```python
from build123d import *

# Parameters (mm, degrees)
F0_W     = 101.6
F0_H     = 50.8
F1_DEPTH = 25.4
F2_W     = 50.8
F2_H     = 12.7
F4_DEPTH = 25.4
F3_W     = 25.4
F3_H     = 12.7
F5_DEPTH = 19.05
F6_R     = 6.35
F7_DEPTH = 101.6


with BuildPart() as f1:
    # F0 (on Front) → F1 (new body)
    with BuildSketch(Plane.XZ):
        Rectangle(F0_W, F0_H)
    extrude(amount=F1_DEPTH)

    # F2 (on face) → F4 (cut)
    with BuildSketch(Plane.XZ.offset(25.4)):
        with Locations((0.033422, 19.05)):
            Rectangle(F2_W, F2_H)
    extrude(amount=-F4_DEPTH, mode=Mode.SUBTRACT)

    # F3 (on face) → F5 (cut)
    with BuildSketch(Plane.YZ.offset(50.8)):
        with Locations((-12.7, -19.05)):
            Rectangle(F3_W, F3_H)
    extrude(amount=-F5_DEPTH, mode=Mode.SUBTRACT)

    # F6 (on face) → F7 (cut)
    with BuildSketch(Plane.YZ.offset(50.8)):
        with Locations((-12.7, 0)):
            Circle(F6_R)
    extrude(amount=-F7_DEPTH, mode=Mode.SUBTRACT)


solid = f1.part
```
Here's how the part is built. I have some questions about the finished solid (model axes, mm). A direction names the side the tool comes from. Coordinates: 2 decimals unless noted, no trailing zeros. Order: outer loops, then holes, each group sorted by start corner. A loop starts at its lowest first (then second) coordinate and runs counter-clockwise, first axis right, second up.
Item 1: Thinking about a two-plate mould opening in X: for faces 1 (the face through (0, -13, 12.7)), 2 (the face through (-50.8, -15.3, -6)), 3 (the face through (0.711, -6.643, 1.907)), 4 (the face through (-25.367, -13, 19)), which applies, pulls with the +X half, pulls with the -X half, needs draft (parallel to the pull), parting line crosses it, or undercut?
Response values:
face 1: undercut
face 2: pulls with the -X half
face 3: needs draft
face 4: undercut
Item 2: Which directions (+Z, -Z, +X, -X, +Y, -Y) give clear straight access to the entire face, cutting with the end or side of a thin tool? Please do faces 5 (the face through (41, -13, -12.7)), 6 (the face through (25.433, -13, 19)), 7 (the face through (50.8, -15.3, 6.1)).
Response values:
face 5: -Z, +X, +Y, -Y
face 6: +Z, +Y, -Y
face 7: +Z, -Z, +X, +Y, -Y
Item 3: If we section it at C-C, the plane x = 36.5: List the corners of the cut face in (y, z) for me, then the cut area to 3 significant figures.
Response values:
outline: (-25.4, -12.7) - (0, -12.7) - (0, 25.4) - (-25.4, 25.4) - close; hole circle Ø12.7 at (-12.7, 0)
area: 841 mm2
Item 4: If we section it at D-D, the plane y = -4.75: List the corners of the cut face in (x, z) for me.
Response values:
outline: (-50.8, -25.4) - (31.75, -25.4) - (31.75, -12.7) - (50.8, -12.7) - (50.8, 25.4) - (25.43, 25.4) - (25.43, 12.7) - (-25.37, 12.7) - (-25.37, 25.4) - (-50.8, 25.4) - close
Item 5: I'm going to push a flat-ended pin straight in: pin 1 Ø7.5 at (x, y) = (-3.5, -14.5) entering from +Z. Where does the tip first touch, or does it pass through?
Response values:
pin 1: stops at z = 12.7
Item 6: If we section it at A-A, the plane y = -12.7: List the corners of the cut face in (x, z) for me.
Response values:
outline: (-50.8, -25.4) - (31.75, -25.4) - (31.75, -12.7) - (50.8, -12.7) - (50.8, -6.35) - (-50.8, -6.35) - close; (-50.8, 6.35) - (50.8, 6.35) - (50.8, 25.4) - (25.43, 25.4) - (25.43, 12.7) - (-25.37, 12.7) - (-25.37, 25.4) - (-50.8, 25.4) - close
Item 7: If we section it at B-B, the plane z = 19: List the corners of the cut face in (x, y) for me, then the cut area to 3 significant figures.
Response values:
outline: (-50.8, -25.4) - (-25.37, -25.4) - (-25.37, 0) - (-50.8, 0) - close; (25.43, -25.4) - (50.8, -25.4) - (50.8, 0) - (25.43, 0) - close
area: 1,290 mm2
Item 8: I need wall thicknesses on probe 1 along Z at (x, y) = (-38.5, -13); probe 2 along X at (y, z) = (-23.5, 13); probe 3 along Z at (x, y) = (21.5, -12.7). Which ranges of each line are inside material? Lowest first, please.
Response values:
probe 1: z = -25.4 to -6.34, 6.34 to 25.4
probe 2: x = -50.8 to -25.37, 25.43 to 50.8
probe 3: z = -25.4 to -6.35, 6.35 to 12.7
